Geometry: final body of the model. Coordinates: model frame, mm. Round coordinates to 2 decimals unless told otherwise and drop trailing zeros. Loops run counter-clockwise (first coordinate to the right, second up) from the corner with the lowest first, then second, coordinate; pieces in that order, holes last. Notation, with made-up numbers: (25.5, 9.25) -> (73.5, 9.25) arc R22 ccw to (73.5, 37.25) -> close; hole circle Ø6 at (3.5, 29.25). An arc over 180 degrees is marked (long way). Answer in a Markdown table with one row per item.
Autodesk Inventor part; units mm, degrees
ref_plane "YZ Plane" through (0, 0, 0) normal (1, 0, 0) x (0, 1, 0)
ref_plane "XZ Plane" through (0, 0, 0) normal (0, 1, 0) x (-1, 0, 0)
ref_plane "XY Plane" through (0, 0, 0) normal (0, 0, 1) x (1, 0, 0)
sketch "Sketch1" plane through (0, 0, 0) normal (0, 1, 0) x (-1, 0, 0)
  line L0 (47.625, 44.45) -> (-47.625, 44.45)
  line L1 (-47.625, 44.45) -> (-47.625, -44.45)
  line L2 (-47.625, -44.45) -> (47.625, -44.45)
  line L3 (47.625, -44.45) -> (47.625, 44.45)
  line L4 (47.625, 0) -> (-47.625, 0)
  line L5 (0, -44.45) -> (0, 44.45)
  point P0 (0, 0)
  point P1 (0, 0)
  dimension "d0" = 95.25
  dimension "d1" = 88.9
extrude "Extrusion1" add sketch "Sketch1" along normal blind 3.175
sketch "Sketch2" plane through (0, 3.175, 0) normal (0, 1, 0) x (1, 0, 0)
  line L0 (47.625, 44.45) -> (-47.625, 44.45)
  line L1 (-47.625, -44.45) -> (47.625, -44.45)
  line L2 (47.625, 44.45) -> (44.45, 44.45)
  line L3 (44.45, 44.45) -> (44.45, -44.45)
  line L4 (44.45, -44.45) -> (47.625, -44.45)
  line L5 (47.625, -44.45) -> (47.625, 44.45)
  line L6 (-47.625, 44.45) -> (-47.625, -44.45)
  line L7 (-47.625, 44.45) -> (-44.45, 44.45)
  line L8 (-44.45, 44.45) -> (-44.45, -44.45)
  line L9 (-44.45, -44.45) -> (-47.625, -44.45)
  line L10 (-47.625, -44.45) -> (-47.625, 44.45)
  point P0 (0, 0)
  point P1 (-44.45, -44.45)
  point P2 (-44.45, 44.45)
  dimension "d4" = 3.175
extrude "Extrusion2" add sketch "Sketch2" along normal blind 73.025 contours L5 L1 L3 L0 | L8 L1 L6 L0
fillet "Fillet1" radius 3.175 4 edges at (47.625, 0, 0) (44.45, 3.175, 0) (-47.625, 0, 0) (-44.45, 3.175, 0)
fillet "Fillet2" radius 25.4 4 edges at (46.0375, 76.2, -44.45) (-46.0375, 76.2, -44.45) (-46.0375, 76.2, 44.45) (46.0375, 76.2, 44.45)
sketch "Sketch3" plane through (47.625, 3.175, 44.45) normal (1, 0, 0) x (0, 0, -1)
  circle A0 centre (69.85, 57.15) radius 3.175
  circle A1 centre (69.85, 31.75) radius 3.175
  line L0 (88.9, 0) -> (88.9, 47.625)
  line L1 (44.45, -3.175) -> (44.45, 73.025)
  line L2 (25.4, 73.025) -> (63.5, 73.025)
  circle A2 centre (19.05, 57.15) radius 3.175
  circle A3 centre (19.05, 31.75) radius 3.175
  circle A4 centre (44.45, 38.1) radius 6.35
  dimension "d10" = 6.35
  dimension "d11" = 19.05
  dimension "d12" = 15.875
  dimension "d13" = 25.4
  dimension "d14" = 19.05
  dimension "d15" = 12.7
  dimension "d16" = 6.35
hole "Hole1" at (47.625, 60.325, 25.4) at (47.625, 60.325, -25.4) at (47.625, 34.925, 25.4) at (47.625, 34.925, -25.4) direction (-1, 0, 0) diameter 6.35 end through all
hole "Hole2" at (47.625, 41.275, 0) direction (-1, 0, 0) diameter 12.7 end through all
sketch "Sketch4" plane through (0, 0, 0) normal (0, -1, 0) x (1, 0, 0)
  circle A0 centre (0, 0) radius 6.35
  dimension "d31" = 12.7
extrude "Extrusion3" add sketch "Sketch4" along normal blind 165.1
properties part number "Saddle_Bracket" material "Steel, Galvanized"
Item 1: Section query A-A, the plane y = 25. Output: boundary loops of the cut face in (x, z) (3 decimals).
Ans:
| item | result |
|---|---|
| outline | (-47.625, -44.45) -> (-44.45, -44.45) -> (-44.45, 44.45) -> (-47.625, 44.45) -> close; (44.45, -44.45) -> (47.625, -44.45) -> (47.625, 44.45) -> (44.45, 44.45) -> close |
Item 2: Section query C-C, the plane z = 25.4. Output: boundary loops of the cut face in (x, y) (3 decimals).
Ans:
| item | result |
|---|---|
| outline | (-47.625, 3.175) arc R3.175 ccw to (-44.45, 0) -> (44.45, 0) arc R3.175 ccw to (47.625, 3.175) -> (47.625, 31.75) -> (44.45, 31.75) -> (44.45, 6.35) arc R3.175 cw to (41.275, 3.175) -> (-41.275, 3.175) arc R3.175 cw to (-44.45, 6.35) -> (-44.45, 31.75) -> (-47.625, 31.75) -> close; (-47.625, 38.1) -> (-44.45, 38.1) -> (-44.45, 57.15) -> (-47.625, 57.15) -> close; (-47.625, 63.5) -> (-44.45, 63.5) -> (-44.45, 75.393) -> (-47.625, 75.393) -> close; (44.45, 38.1) -> (47.625, 38.1) -> (47.625, 57.15) -> (44.45, 57.15) -> close; (44.45, 63.5) -> (47.625, 63.5) -> (47.625, 75.393) -> (44.45, 75.393) -> close |
Item 3: Section query D-D, the plane x = 0. Output: boundary loops of the cut face in (y, z) (3 decimals).
Ans:
| item | result |
|---|---|
| outline | (-165.1, -6.35) -> (0, -6.35) -> (0, -44.45) -> (3.175, -44.45) -> (3.175, 44.45) -> (0, 44.45) -> (0, 6.35) -> (-165.1, 6.35) -> close |
Item 4: Section query B-B, the plane z = -3. Output: boundary loops of the cut face in (x, y) (3 decimals).
Ans:
| item | result |
|---|---|
| outline | (-47.625, 3.175) arc R3.175 ccw to (-44.45, 0) -> (-5.597, 0) -> (-5.597, -165.1) -> (5.597, -165.1) -> (5.597, 0) -> (44.45, 0) arc R3.175 ccw to (47.625, 3.175) -> (47.625, 35.678) -> (44.45, 35.678) -> (44.45, 6.35) arc R3.175 cw to (41.275, 3.175) -> (-41.275, 3.175) arc R3.175 cw to (-44.45, 6.35) -> (-44.45, 35.678) -> (-47.625, 35.678) -> close; (-47.625, 46.872) -> (-44.45, 46.872) -> (-44.45, 76.2) -> (-47.625, 76.2) -> close; (44.45, 46.872) -> (47.625, 46.872) -> (47.625, 76.2) -> (44.45, 76.2) -> close |
Item 5: Mould query, pull axis X, two halves, no side actions, for faces 1 (the flat face through (44.45, 33, -1)), 2 (the flat face through (1, 3.175, 1)), 3 (the cylindrical face through (-1.38, -81.39, 6.2)), 4 (the flat face through (-47.625, 31, -1)). Classes: released by +X, released by -X, zero draft, split by the parting line, or undercut.
Ans:
| item | result |
|---|---|
| face 1 | undercut |
| face 2 | undercut |
| face 3 | split by the parting line |
| face 4 | released by -X |
Item 6: First-contact query: P1, Ø5.5, axis at y = 60.325, z = -25.4, coming from the -X side; P2, Ø2, axis at y = -1.5, z = 1, coming from the -X side; P3, Ø5, axis at x = -10.5, z = 29, coming from the +Y side (3 decimals); P4, Ø5, axis at x = 10.5, z = -3, coming from the -Y side. Flat tips, straight axial feed; report the tip coordinate or a pass-through.
Ans:
| item | result |
|---|---|
| P1 | through |
| P2 | x = -6.35 |
| P3 | y = 3.175 |
| P4 | y = 0 |
Item 7: Ray query, L1, parallel to X at y = 62, z = 6.5 (3 decimals); L2, parallel to Y at x = 33, z = -17 (3 decimals); L3, parallel to Y at x = -45.1, z = 25.4. Return the intervals inside material, ascending.
Ans:
| item | result |
|---|---|
| L1 | -47.625 to -44.45, 44.45 to 47.625 |
| L2 | 0 to 3.175 |
| L3 | 0.07 to 31.75, 38.1 to 57.15, 63.5 to 75.39 |
